Source: three-view drawing plus pictorial views. Frame: mm from the lowest corner of the part. Give positions to 0.01 mm unless a question says otherwise; leave off trailing zeros. Loops run counter-clockwise (first coordinate to the right, second up) from the corner with the lowest first, then second, coordinate; pieces in that order, holes last. Notation, with made-up numbers: (34, 22.5) - (57, 22.5) arc R25 ccw to (57, 60.5) - close; hole circle Ø7 at (89.5, -39). An arc over 180 degrees is marked (long way). Put each result on its own line as item: value.
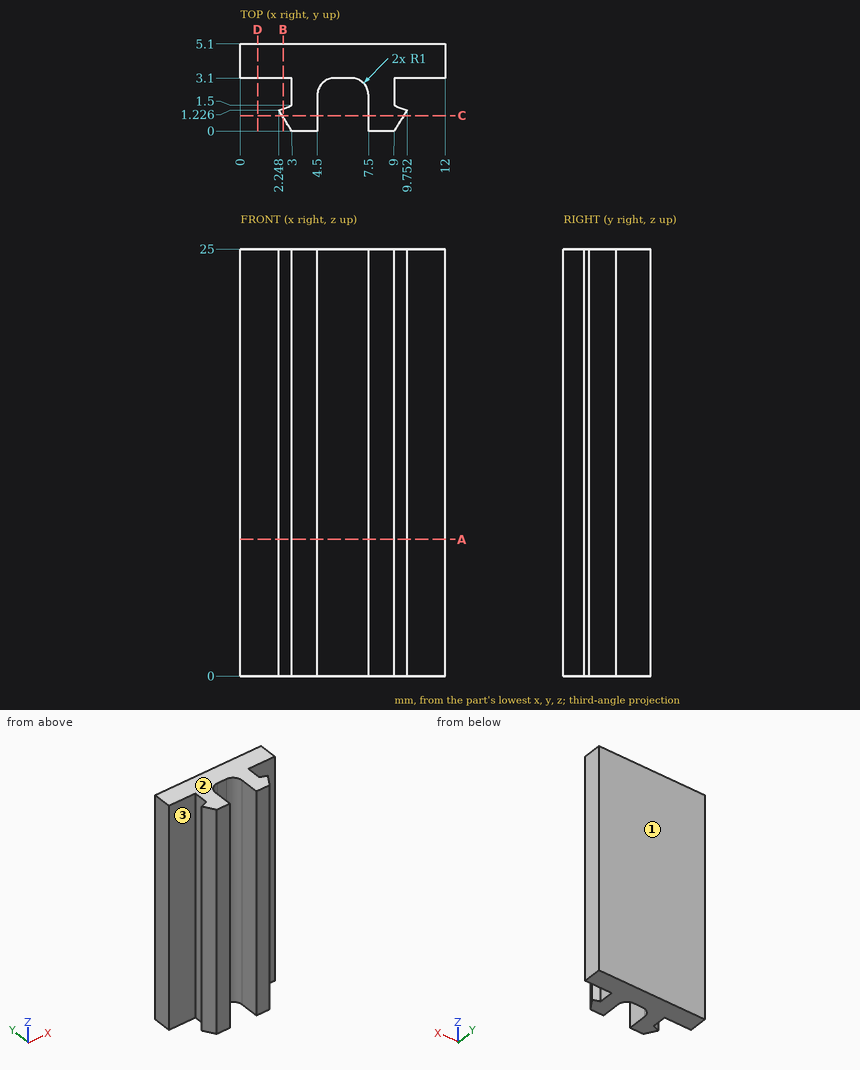
1) Mould query, pull axis Y, two halves, no side actions, for the marked faces 1, 2 and 3. Classes: pulls with the +Y half, pulls with the -Y half, needs draft (parallel to the pull), parting line crosses it, or undercut.
Check result:
face 1: pulls with the +Y half
face 2: needs draft
face 3: undercut
2) Pin query (flat end, axial travel): P1, Ø3, axis at x = 9, z = 6.5, coming from the -Y side; P2, Ø1.1, axis at x = 6, z = 10.5, coming from the -Y side; P3, Ø1.7, axis at y = 1.5, z = 17.5, coming from the +X side; P4, Ø1, axis at y = 1.5, z = 11.5, coming from the -X side. Return the tip coordinate at first contact, or that it passes through.
Check result:
P1: y = 0
P2: y = 3.1
P3: x = 9.75
P4: x = 2.25
3) Section query A-A, the plane z = 8. Output: boundary loops of the cut face in (x, y).
Check result:
outline: (0, 3.1) - (3, 3.1) - (3, 1.5) - (2.25, 1.23) - (3, 0) - (4.5, 0) - (4.5, 2.1) arc R1 cw to (5.5, 3.1) - (6.5, 3.1) arc R1 cw to (7.5, 2.1) - (7.5, 0) - (9, 0) - (9.75, 1.23) - (9, 1.5) - (9, 3.1) - (12, 3.1) - (12, 5.1) - (0, 5.1) - close
4) Section query D-D, the plane x = 1. Output: boundary loops of the cut face in (y, z).
Check result:
outline: (3.1, 0) - (5.1, 0) - (5.1, 25) - (3.1, 25) - close
5) Section query B-B, the plane x = 2.5. Output: boundary loops of the cut face in (y, z) (1 decimal).
Check result:
outline: (0.8, 0) - (1.3, 0) - (1.3, 25) - (0.8, 25) - close; (3.1, 0) - (5.1, 0) - (5.1, 25) - (3.1, 25) - close
6) Section query C-C, the plane y = 0.9. Output: boundary loops of the cut face in (x, z).
Check result:
outline: (2.45, 0) - (4.5, 0) - (4.5, 25) - (2.45, 25) - close; (7.5, 0) - (9.55, 0) - (9.55, 25) - (7.5, 25) - close
7) Material intervals for line 1 along X through (y, z) = (1.6, 18.5); line 2 along X through (y, z) = (3, 12) (1 decimal); line 3 along Y through (x, z) = (1.5, 14.25), sorted ascending. Write a range as [from, to].
Check result:
line 1: [3, 4.5], [7.5, 9]
line 2: [3, 5.1], [6.9, 9]
line 3: [3.1, 5.1]
